from build123d import *

# Parameters (mm, degrees)
SKETCH1_R           = 1.5
BOSS_EXTRUDE1_DEPTH = 1.6
SKETCH2_W           = 2.54
SKETCH2_H           = 1.27
SKETCH2_W_2         = 1.27
SKETCH2_H_2         = 2.54
BOSS_EXTRUDE2_DEPTH = 0.1
SKETCH3_W           = 5
SKETCH3_H           = 2
BOSS_EXTRUDE3_DEPTH = 1


with BuildPart() as part:
    # Sketch1 → Boss-Extrude1 (new body)
    with BuildSketch(Plane(origin=(0, 0, 0), x_dir=(1, 0, 0), z_dir=(0, 1, 0))):
        with BuildLine():
            Line((14.5, 13), (-14.5, 13))
            ThreePointArc((-14.5, 13), (-15.914213562, 12.414213562), (-16.5, 11))
            Line((-16.5, 11), (-16.5, -11))
            ThreePointArc((-16.5, -11), (-15.914213562, -12.414213562), (-14.5, -13))
            Line((-14.5, -13), (14.5, -13))
            ThreePointArc((14.5, -13), (15.914213562, -12.414213562), (16.5, -11))
            Line((16.5, -11), (16.5, 11))
            ThreePointArc((16.5, 11), (15.914213562, 12.414213562), (14.5, 13))
        make_face()
        with Locations(Location((0, -3.5, 0), (0, 0, 270))):
            Circle(SKETCH1_R, mode=Mode.SUBTRACT)
        with Locations(Location((10.5, 4, 0), (0, 0, 270))):
            Circle(SKETCH1_R, mode=Mode.SUBTRACT)
        with Locations(Location((10.5, -9, 0), (0, 0, 270))):
            Circle(SKETCH1_R, mode=Mode.SUBTRACT)
    extrude(amount=BOSS_EXTRUDE1_DEPTH)

    # Sketch2 → Boss-Extrude2 (add)
    with BuildSketch(Plane(origin=(0, 1.6, 0), x_dir=(1, 0, 0), z_dir=(0, 1, 0))):
        with Locations((-13.96, 9.86)):
            Rectangle(SKETCH2_W, SKETCH2_H)
        with Locations((-6.34, 9.86)):
            Rectangle(SKETCH2_W_2, SKETCH2_H_2)
        with Locations((-13.96, 7.32)):
            Rectangle(SKETCH2_W, SKETCH2_H)
        with Locations((-13.96, 4.78)):
            Rectangle(SKETCH2_W, SKETCH2_H)
        with Locations((-13.96, 2.24)):
            Rectangle(SKETCH2_W, SKETCH2_H)
        with Locations((-13.96, -0.3)):
            Rectangle(SKETCH2_W, SKETCH2_H)
        with Locations((-13.96, -2.84)):
            Rectangle(SKETCH2_W, SKETCH2_H)
        with Locations((-13.96, -5.38)):
            Rectangle(SKETCH2_W, SKETCH2_H)
        with Locations((-13.96, -7.92)):
            Rectangle(SKETCH2_W, SKETCH2_H)
        with Locations((-13.96, -10.46)):
            Rectangle(SKETCH2_W, SKETCH2_H)
        with Locations((-4.96, 2.24)):
            Rectangle(SKETCH2_W, SKETCH2_H)
        with Locations((-4.96, -0.3)):
            Rectangle(SKETCH2_W, SKETCH2_H)
        with Locations((-4.96, -2.84)):
            Rectangle(SKETCH2_W, SKETCH2_H)
        with Locations((-4.96, -5.38)):
            Rectangle(SKETCH2_W, SKETCH2_H)
        with Locations((-4.96, -7.92)):
            Rectangle(SKETCH2_W, SKETCH2_H)
        with Locations((-4.96, -10.46)):
            Rectangle(SKETCH2_W, SKETCH2_H)
        with Locations((4.04, 2.24)):
            Rectangle(SKETCH2_W, SKETCH2_H)
        with Locations((4.04, -0.3)):
            Rectangle(SKETCH2_W, SKETCH2_H)
        with Locations((4.04, -2.84)):
            Rectangle(SKETCH2_W, SKETCH2_H)
        with Locations((4.04, -5.38)):
            Rectangle(SKETCH2_W, SKETCH2_H)
        with Locations((4.04, -7.92)):
            Rectangle(SKETCH2_W, SKETCH2_H)
        with Locations((4.04, -10.46)):
            Rectangle(SKETCH2_W, SKETCH2_H)
        with Locations((-3.42, 9.86)):
            Rectangle(SKETCH2_W_2, SKETCH2_H_2)
        with Locations((-0.5, 9.86)):
            Rectangle(SKETCH2_W_2, SKETCH2_H_2)
        with Locations((2.42, 9.86)):
            Rectangle(SKETCH2_W_2, SKETCH2_H_2)
        with Locations((5.34, 9.86)):
            Rectangle(SKETCH2_W_2, SKETCH2_H_2)
        with Locations((8.26, 9.86)):
            Rectangle(SKETCH2_W_2, SKETCH2_H_2)
        with Locations((11.18, 9.86)):
            Rectangle(SKETCH2_W_2, SKETCH2_H_2)
        with Locations((14.1, 9.86)):
            Rectangle(SKETCH2_W_2, SKETCH2_H_2)
    extrude(amount=BOSS_EXTRUDE2_DEPTH)

    # Sketch3 → Boss-Extrude3 (add)
    with BuildSketch(Plane(origin=(0, 1.6, 0), x_dir=(1, 0, 0), z_dir=(0, 1, 0))):
        with Locations((-5.07, 5.05)):
            Rectangle(SKETCH3_W, SKETCH3_H)
        with Locations((2.55, 5.05)):
            Rectangle(SKETCH3_W, SKETCH3_H)
    extrude(amount=BOSS_EXTRUDE3_DEPTH)


solid = part.part
Build history of the part. All positions in model axes, mm. A direction names the side the tool comes from. Round coordinates to 2 decimals unless told otherwise and drop trailing zeros. Write each loop counter-clockwise with the first axis right and the second up, starting at its lowest first coordinate (ties: lowest second). Pieces come first, ordered by that corner, then holes. Notation, with made-up numbers: M -5.75,12.25 L -0.75,12.25 A11 cw -0.75,22.25 Z; hole C -15,35.25 d6. An arc over 180 degrees is marked long. Answer in a Markdown table with one row per item.
1. Flat gauge pins, fed straight in: P1, Ø1.5, axis at x = 11.5, y = 2.5, coming from the +Z side; P2, Ø1, axis at x = -13.5, z = -2.5, coming from the +Y side. Where does each tip first touch, or does it go through?
Geometry check:
| item | result |
|---|---|
| P1 | through |
| P2 | y = 1.7 |
2. Saw through at B-B (z = 9). List the corners of the cut face in (x, y).
Geometry check:
| item | result |
|---|---|
| outline | M -16.5,0 L 9,0 L 9,1.6 L -16.5,1.6 Z; M 12,0 L 16.5,0 L 16.5,1.6 L 12,1.6 Z |
3. Mould opens along X. For faces 1 (the face through (-14, 1.7, 0)), 2 (the face through (-16.5, 1, 0)), 3 (the face through (10.95, 0.79, -2.57)) say: +X half, -X half, draft (parallel to the pull), parting line (faces both ways), or undercut.
Geometry check:
| item | result |
|---|---|
| face 1 | draft |
| face 2 | -X half |
| face 3 | undercut |
4. Saw through at A-A (y = 0.45). List the corners of the cut face in (x, z), and give its area (3 significant figures).
Geometry check:
| item | result |
|---|---|
| outline | M -16.5,-11 A2 ccw -14.5,-13 L 14.5,-13 A2 ccw 16.5,-11 L 16.5,11 A2 ccw 14.5,13 L -14.5,13 A2 ccw -16.5,11 Z; hole C 0,3.5 d3; hole C 10.5,-4 d3; hole C 10.5,9 d3 |
| area | 833 mm2 |
5. Which spindle directions (+Z, -Z, +X, -X, +Y, -Y) get a long thin tool onto all of the face, cutting with end or side? Do faces 4 (the face through (14, 1.7, -10)), 5 (the face through (2, 1.7, -10)), 6 (the face through (4, 1.7, 10)). Say none if no direction does.
Geometry check:
| item | result |
|---|---|
| face 4 | +Z, -Z, +X, -X, +Y |
| face 5 | -Z, +X, -X, +Y |
| face 6 | +Z, +X, -X, +Y |
6. Saw through at C-C (x = 9.5). List the corners of the cut face in (y, z), and give its area (3 significant figures).
Geometry check:
| item | result |
|---|---|
| outline | M 0,-13 L 1.6,-13 L 1.6,-5.12 L 0,-5.12 Z; M 0,-2.88 L 1.6,-2.88 L 1.6,7.88 L 0,7.88 Z; M 0,10.12 L 1.6,10.12 L 1.6,13 L 0,13 Z |
| area | 34.4 mm2 |
7. Probe L1, parallel to X at y = 0.7, z = -4; L2, parallel to X at y = 0.6, z = 3.5; L3, parallel to Y at x = 12.5, z = -1.75. List the from-to ranges inside material, lowest first. Write a range as [from, to].
Geometry check:
| item | result |
|---|---|
| L1 | [-16.5, 9], [12, 16.5] |
| L2 | [-16.5, -1.5], [1.5, 16.5] |
| L3 | [0, 1.6] |
